Design review of the part built by this model. Coordinates are the model's own, in mm. Coordinates: 2 decimals unless noted, no trailing zeros. Order: outer loops, then holes, each group sorted by start corner. A loop starts at its lowest first (then second) coordinate and runs counter-clockwise, first axis right, second up. Notation, with made-up numbers: M 50,-10 L 107,-10 A18 ccw 107,16 Z; hole C 20.5,84.25 d5. An arc over 180 degrees is marked long. Answer in a Markdown table with one row per item.
from build123d import *

# Parameters (mm, degrees)
F0_W     = 30
F0_H     = 25
F1_DEPTH = 3
F2_R     = 2
F3_R     = 5
F4_DEPTH = 3
F5_R     = 2
F6_DEPTH = 3


with BuildPart() as f1:
    # F0 (on Top) → F1 (new body)
    with BuildSketch(Plane.XY):
        Rectangle(F0_W, F0_H)
    extrude(amount=F1_DEPTH)

    # F2
    f2_edges = [f1.edges().sort_by_distance(p)[0] for p in [
        (15, 12.5, 1.5),
        (-15, 12.5, 1.5),
        (-15, -12.5, 1.5),
        (15, -12.5, 1.5),
    ]]
    fillet(f2_edges, radius=F2_R)

    # F3 (on face) → F4 (cut)
    with BuildSketch(Plane.XY.offset(3)):
        Circle(F3_R)
    extrude(amount=-F4_DEPTH, mode=Mode.SUBTRACT)

    # F5 (on face) → F6 (cut)
    with BuildSketch(Plane.XY.offset(3)):
        with Locations((-11.434802, 9.066023)):
            Circle(F5_R)
        with Locations((11.434802, 9.066023)):
            Circle(F5_R)
        with Locations((-11.434802, -9.066023)):
            Circle(F5_R)
        with Locations((11.434802, -9.066023)):
            Circle(F5_R)
    extrude(amount=-F6_DEPTH, mode=Mode.SUBTRACT)


solid = f1.part
(1) Add section B-B, the plane x = 0. Give the boundary of the cut face in (y, z).
Return value:
| item | result |
|---|---|
| outline | M -12.5,0 L -5,0 L -5,3 L -12.5,3 Z; M 5,0 L 12.5,0 L 12.5,3 L 5,3 Z |
(2) Add section A-A, the plane y = 0. Give the boundary of the cut face in (x, z).
Return value:
| item | result |
|---|---|
| outline | M -15,0 L -5,0 L -5,3 L -15,3 Z; M 5,0 L 15,0 L 15,3 L 5,3 Z |
(3) Insertion check: pin 1 Ø6 at (x, y) = (0, 0) entering from +Z; pin 2 Ø5 at (x, y) = (-2, 3) entering from +Z. Each pin has a flat end and moves straight along its axis. Give the tip position at first contact, or say it passes through.
Return value:
| item | result |
|---|---|
| pin 1 | passes through |
| pin 2 | stops at z = 3 |
(4) For line 1 along X through (y, z) = (-9, 0.25); line 2 along Y through (x, z) = (-11.25, 0.4); line 3 along Y through (x, z) = (10.5, 2.75), list the stretches that pass through material, from the lowest coordinate up. Write a range as from..to.
Return value:
| item | result |
|---|---|
| line 1 | x = -15..-13.43, -9.44..9.44, 13.43..15 |
| line 2 | y = -12.5..-11.06, -7.07..7.07, 11.06..12.5 |
| line 3 | y = -12.5..-10.83, -7.3..7.3, 10.83..12.5 |
(5) Add section D-D, the plane x = -11. Give the boundary of the cut face in (y, z), and give its area (3 significant figures).
Return value:
| item | result |
|---|---|
| outline | M -12.5,0 L -11.02,0 L -11.02,3 L -12.5,3 Z; M -7.11,0 L 7.11,0 L 7.11,3 L -7.11,3 Z; M 11.02,0 L 12.5,0 L 12.5,3 L 11.02,3 Z |
| area | 51.6 mm2 |
(6) Draft analysis for pull direction Y (two halves, no side actions). For faces 1 (the cylindrical face through (12.51, -7.38, 1.52)), 2 (the flat face through (0, 6, 3)), 3 (the flat face through (0, -12.5, 1)), state which applies: pulls with the +Y half, pulls with the -Y half, needs draft (parallel to the pull), parting line crosses it, or undercut.
Return value:
| item | result |
|---|---|
| face 1 | undercut |
| face 2 | needs draft |
| face 3 | pulls with the -Y half |
(7) Add section C-C, the plane z = 0.9. Give the boundary of the cut face in (x, y).
Return value:
| item | result |
|---|---|
| outline | M -15,-10.5 A2 ccw -13,-12.5 L 13,-12.5 A2 ccw 15,-10.5 L 15,10.5 A2 ccw 13,12.5 L -13,12.5 A2 ccw -15,10.5 Z; hole C -11.43,-9.07 d4; hole C -11.43,9.07 d4; hole C 0,0 d10; hole C 11.43,-9.07 d4; hole C 11.43,9.07 d4 |
